```python
from build123d import *

# Parameters (mm, degrees)
SKETCH1_R               = 9.6
BOSS_EXTRUDE1_DEPTH     = 0.8
CUT_EXTRUDE4_START      = 0.8
SKETCH3_R               = 2
SKETCH3_W               = 1
SKETCH3_H               = 1
CUT_EXTRUDE4_DEPTH      = 1.8
CUT_EXTRUDE4_DEPTH_BACK = 1.8


with BuildPart() as part:
    # Sketch1 → Boss-Extrude1 (new body)
    with BuildSketch(Plane.XY):
        Circle(SKETCH1_R)
    extrude(amount=BOSS_EXTRUDE1_DEPTH)

    # Sketch3 → Cut-Extrude4 (cut, two sides)
    with BuildSketch(Plane.XY.offset(CUT_EXTRUDE4_START)) as cut_extrude4_sk:
        Circle(SKETCH3_R)
        with Locations((-4.5, 0)):
            Rectangle(SKETCH3_W, SKETCH3_H)
        with Locations((4.5, 0)):
            Rectangle(SKETCH3_W, SKETCH3_H)
    extrude(amount=CUT_EXTRUDE4_DEPTH, mode=Mode.SUBTRACT)
    extrude(cut_extrude4_sk.sketch, amount=-CUT_EXTRUDE4_DEPTH_BACK, mode=Mode.SUBTRACT)


solid = part.part
```
Part model, mm, in its own coordinate system. Give positions to 0.01 mm unless a question says otherwise; leave off trailing zeros. Order: outer loops, then holes, each group sorted by start corner. A loop starts at its lowest first (then second) coordinate and runs counter-clockwise, first axis right, second up. Notation, with made-up numbers: M -39,35 L -15,35 A13 ccw -15,43 Z; hole C 55.5,32 d5. An arc over 180 degrees is marked long. Use a Markdown table: item, result. Add a question column.
(1) Saw through at B-B, the plane y = 0. Give the cut face in (x, z), and give its area (3 significant figures).
(2) Saw through at D-D, the plane x = -4.5. Give the cut face in (y, z).
(3) Saw through at A-A, the plane x = 0. Give the cut face in (y, z).
(4) Mould opens along X. For faces 1 (the face through (5.161, 8.095, 0.394)), 2 (the face through (-0.434, -1.952, 0.406)), 3 (the face through (-0.1, 2.3, 0)) say: +X half, -X half, draft (parallel to the pull), parting line (faces both ways), or undercut.
(5) Drop a flat-ended pin along its axis: P1, Ø5, axis at x = 0, y = 0, coming from the +Z side. Give the stop position or say it passes through.
(6) Probe line 1 along Y through (x, z) = (0, 0.6); line 2 along X through (y, z) = (1.75, 0.3); line 3 along Y through (x, z) = (1.5, 0.35). List the from-to ranges inside material, lowest first. Write a range as [from, to].
(7) Saw through at C-C, the plane z = 0.5. Give the cut face in (x, y), and give its area (3 significant figures).
Answer key:
| question | item | result |
|---|---|---|
| 1 | outline | M -9.6,0 L -5,0 L -5,0.8 L -9.6,0.8 Z; M -4,0 L -2,0 L -2,0.8 L -4,0.8 Z; M 2,0 L 4,0 L 4,0.8 L 2,0.8 Z; M 5,0 L 9.6,0 L 9.6,0.8 L 5,0.8 Z |
| 1 | area | 10.6 mm^2 |
| 2 | outline | M -8.48,0 L -0.5,0 L -0.5,0.8 L -8.48,0.8 Z; M 0.5,0 L 8.48,0 L 8.48,0.8 L 0.5,0.8 Z |
| 3 | outline | M -9.6,0 L -2,0 L -2,0.8 L -9.6,0.8 Z; M 2,0 L 9.6,0 L 9.6,0.8 L 2,0.8 Z |
| 4 | face 1 | parting line |
| 4 | face 2 | undercut |
| 4 | face 3 | draft |
| 5 | P1 | z = 0.8 |
| 6 | line 1 | [-9.6, -2], [2, 9.6] |
| 6 | line 2 | [-9.44, -0.97], [0.97, 9.44] |
| 6 | line 3 | [-9.48, -1.32], [1.32, 9.48] |
| 7 | outline | C 0,0 d19.2; hole M -5,-0.5 L -4,-0.5 L -4,0.5 L -5,0.5 Z; hole C 0,0 d4; hole M 4,-0.5 L 5,-0.5 L 5,0.5 L 4,0.5 Z |
| 7 | area | 275 mm^2 |
